from build123d import *


with BuildPart() as part:
    # Sketch1 → Revolve1 (revolve)
    with BuildSketch(Plane.XY, mode=Mode.PRIVATE) as revolve1_sk:
        with BuildLine():
            Line((0, -3.81), (0, 0))
            Line((0, 0), (24.892, 0))
            ThreePointArc((24.892, 0), (24.734418278, -0.418684593), (24.339884132, -0.629567487))
            Line((24.339884132, -0.629567487), (19.475316237, -1.27))
            Line((19.475316237, -1.27), (4.318, -1.27))
            ThreePointArc((4.318, -1.27), (1.921768792, -1.957230068), (0.254, -3.81))
            Line((0.254, -3.81), (0, -3.81))
        make_face()
    revolve(revolve1_sk.sketch.rotate(Axis((0, 0, 0), (1, 0, 0)), 270), axis=Axis((0, 0, 0), (1, 0, 0)))


solid = part.part
Part model, mm, in its own coordinate system. A direction names the side the tool comes from. Round coordinates to 2 decimals unless told otherwise and drop trailing zeros. Write each loop counter-clockwise with the first axis right and the second up, starting at its lowest first coordinate (ties: lowest second). Pieces come first, ordered by that corner, then holes. Notation, with made-up numbers: M -19.5,-33.75 L 7.5,-33.75 A7 cw 7.5,-25.75 Z; hole C -19,75.5 d4. An arc over 180 degrees is marked long. Return JSON: item names as keys, results as strings. Group by question number.
(1) Saw through at C-C on x = 5.25. Write the cut outline in (y, z), then the cut area to 3 significant figures.
(2) Saw through at A-A on z = 0. Write the cut outline in (x, y) (3 decimals), then the cut area to 3 significant figures.
(3) Drill centre lines: probe 1 along Z at (x, y) = (15.75, -0.5); probe 2 along Y at (x, z) = (7, -1); probe 3 along X at (y, z) = (0.5, -2.5). Where is each one in solid material? Low to high.
(4) Which spindle directions (+Z, -Z, +X, -X, +Y, -Y) get a long thin tool onto all of the face, cutting with end or side? Do faces 1 (the face through (11.79, -1.26, -0.17)), 2 (the face through (0, 0, 0)). Say none if no direction does.
(5) Pin check, flat tips, straight feed: pin 1 Ø2 at (x, y) = (8.5, -1.5) entering from -Z; pin 2 Ø4 at (x, y) = (20, 2) entering from -Z; pin 3 Ø1.5 at (x, z) = (13.5, 0) entering from -Y; pin 4 Ø3 at (x, z) = (18, 3) entering from +Y. Stop position of each tip, or through.
Returned:
{
 "1": {"outline": "C 0,0 d2.54", "area": "5.07 mm²"},
 "2": {"outline": "M 0,-3.81 L 0.254,-3.81 A4.521 cw 4.318,-1.27 L 19.475,-1.27 L 24.34,-0.63 A0.635 ccw 24.34,0.63 L 19.475,1.27 L 4.318,1.27 A4.521 cw 0.254,3.81 L 0,3.81 Z", "area": "66.4 mm²"},
 "3": {"probe 1": "-1.17 to 1.17", "probe 2": "-0.78 to 0.78", "probe 3": "0 to 1.17"},
 "4": {"face 1": "+X", "face 2": "+Z, -Z, -X, +Y, -Y"},
 "5": {"pin 1": "z = -1.17", "pin 2": "z = -1.27", "pin 3": "y = -1.27", "pin 4": "through"}
}
